Design review of the part built by this model. Coordinates are the model's own, in mm. Face numbers are marked on the shaded views. A direction names the side the tool comes from. Coordinates: 2 decimals unless noted, no trailing zeros. Write each loop counter-clockwise with the first axis right and the second up, starting at its lowest first coordinate (ties: lowest second). Pieces come first, ordered by that corner, then holes.
Q1. Add section C-C, the plane z = -6.75. Give the boundary of the cut face in (x, y).
Q2. The part is to be moulded in two halves that separate along X. For the marked faces 1, 2, 3 and 4, say which applies: +X half, -X half, draft (parallel to the pull), parting line (faces both ways), or undercut.
Q3. Clearance check with flat-ended pins moving along their axes: pin 1 Ø5 at (y, z) = (9, 1.5) entering from -X; pin 2 Ø0.7 at (x, z) = (0, -7.5) entering from +Y; pin 3 Ø8 at (x, z) = (-1.5, 6) entering from -Y; pin 4 Ø3 at (x, y) = (-4.5, 5.5) entering from -Z. State where each tip first meets the part, or that it passes through.
Q4. Machinability: for the marked faces 5, 6 and 7, which of the approach directions +Z, -Z, +X, -X, +Y, -Y give a long, thin tool a straight path to every point of the face, cutting with its end or side? Answer none if there is none.
Q5. To check wall thickness, follow probe 1 along Z at (x, y) = (0, 6.5); probe 2 along X at (y, z) = (5.25, 0); probe 3 along X at (y, z) = (11, 0) (3 decimals). State the ranges of each line that lie inside material, in increasing order.
Q6. Add section B-B, the plane x = 0. Give the boundary of the cut face in (y, z), plus the area to 3 significant figures.
Q7. Add section D-D, the plane y = 3. Give the boundary of the cut face in (x, z) (3 decimals), plus the area to 3 significant figures.
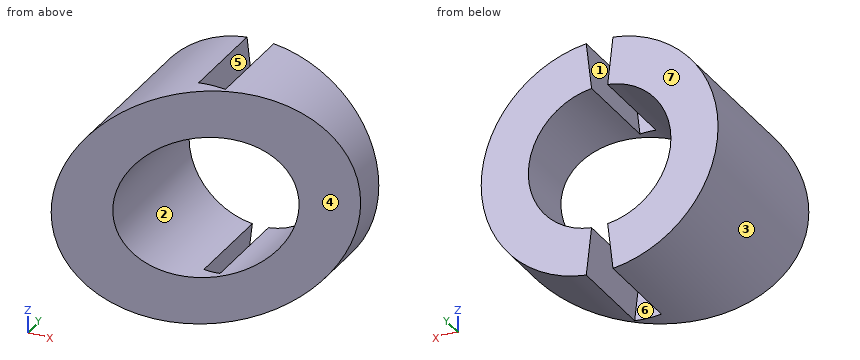
from build123d import *

# Parameters (mm, degrees)
SKETCH1_R           = 10.05
SKETCH1_R_2         = 6.05
BOSS_EXTRUDE1_DEPTH = 15
CUT_EXTRUDE2_DEPTH  = 8
CUT_EXTRUDE3_DEPTH  = 15


with BuildPart() as part:
    # Sketch1 → Boss-Extrude1 (new body)
    with BuildSketch(Plane(origin=(0, 0, 0), x_dir=(1, 0, 0), z_dir=(0, 1, 0))):
        with Locations(Location((0, 0, 0), (0, 0, 270))):
            Circle(SKETCH1_R)
        with Locations(Location((0, 0, 0), (0, 0, 270))):
            Circle(SKETCH1_R_2, mode=Mode.SUBTRACT)
    extrude(amount=BOSS_EXTRUDE1_DEPTH)

    # Sketch6 → Cut-Extrude2 (cut)
    with BuildSketch(Plane(origin=(0, 15, 0), x_dir=(1, 0, 0), z_dir=(0, 1, 0))):
        Polygon((-0.637272671, 5.61077026), (0.637272671, 5.61077026), (1.215708589, 10.703521268), (-1.215708589, 10.703521268), align=None)
        Polygon((-0.637272671, -5.61077026), (-1.215708589, -10.703521268), (1.215708589, -10.703521268), (0.637272671, -5.61077026), align=None)
    extrude(amount=-CUT_EXTRUDE2_DEPTH, mode=Mode.SUBTRACT)

    # Sketch3 → Cut-Extrude3 (cut, symmetric)
    with BuildSketch(Plane.XY):
        Polygon((-10.05, 0), (10.05, 12), (10.05, 0), align=None)
    extrude(amount=CUT_EXTRUDE3_DEPTH, both=True, mode=Mode.SUBTRACT)


solid = part.part
Here are the results:
1. outline: (-7.45, 1.55) - (7.45, 10.45) - (7.45, 15) - (0.77, 15) - (0.77, 7) - (-0.77, 7) - (-0.77, 15) - (-7.45, 15) - close
2. face 1: undercut
2. face 2: undercut
2. face 3: parting line
2. face 4: +X half
3. pin 1: stops at x = -10.05
3. pin 2: stops at y = 7
3. pin 3: stops at y = 2.72
3. pin 4: stops at z = -9.59
4. face 5: +Z, +Y
4. face 6: -Z, +Y
4. face 7: +Z, -Z, +X, -X, +Y
5. probe 1: z = -10.05 to -6.05, 6.05 to 10.05
5. probe 2: x = -10.05 to -6.05
5. probe 3: x = -10.05 to -6.05, 6.05 to 8.375
6. outline: (6, -10.05) - (7, -10.05) - (7, -6.05) - (6, -6.05) - close; (6, 6.05) - (7, 6.05) - (7, 10.05) - (6, 10.05) - close
6. area: 8.00 mm2
7. outline: (-5.025, -8.704) - (-5.025, -3.369) arc R6.05 cw to (-5.025, 3.369) - (-5.025, 8.704) arc R10.05 ccw to start
7. area: 57.3 mm2
